```python
from build123d import *

# Parameters (mm, degrees)
SKETCH1_W           = 234
SKETCH1_H           = 178
BOSS_EXTRUDE1_DEPTH = 3
BOSS_EXTRUDE1_TAPER = 9
SKETCH2_R           = 3.5
SKETCH2_R_2         = 1.4
BOSS_EXTRUDE2_DEPTH = 5
SKETCH3_R           = 1.6
CUT_EXTRUDE1_DEPTH  = 3
CHAMFER1_SIZE       = 2


with BuildPart() as part:
    # Sketch1 → Boss-Extrude1 (new body)
    with BuildSketch(Plane(origin=(0, 0, 0), x_dir=(0, 0, -1), z_dir=(1, 0, 0))):
        Rectangle(SKETCH1_W, SKETCH1_H)
    extrude(amount=BOSS_EXTRUDE1_DEPTH, taper=BOSS_EXTRUDE1_TAPER)

    # Sketch2 → Boss-Extrude2 (add)
    with BuildSketch(Plane(origin=(3, 0, 0), x_dir=(0, 0, -1), z_dir=(1, 0, 0))):
        with Locations((-92.524846679, -22.175153321)):
            Circle(SKETCH2_R)
        with Locations((-92.524846679, -22.175153321)):
            Circle(SKETCH2_R_2, mode=Mode.SUBTRACT)
        with Locations((58.475153321, 62.224846679)):
            Circle(SKETCH2_R)
        with Locations((58.475153321, 62.224846679)):
            Circle(SKETCH2_R_2, mode=Mode.SUBTRACT)
        with Locations((-81.563741741, 52.524846679)):
            Circle(SKETCH2_R)
        with Locations((-81.563741741, 52.524846679)):
            Circle(SKETCH2_R_2, mode=Mode.SUBTRACT)
        with Locations((17.436258259, 52.524846679)):
            Circle(SKETCH2_R)
        with Locations((17.436258259, 52.524846679)):
            Circle(SKETCH2_R_2, mode=Mode.SUBTRACT)
        with Locations((42.436258259, 47.531127093)):
            Circle(SKETCH2_R)
        with Locations((42.436258259, 47.531127093)):
            Circle(SKETCH2_R_2, mode=Mode.SUBTRACT)
        with Locations((68.436258259, 47.531127093)):
            Circle(SKETCH2_R)
        with Locations((68.436258259, 47.531127093)):
            Circle(SKETCH2_R_2, mode=Mode.SUBTRACT)
        with Locations((42.436258259, -10.468872907)):
            Circle(SKETCH2_R)
        with Locations((42.436258259, -10.468872907)):
            Circle(SKETCH2_R_2, mode=Mode.SUBTRACT)
        with Locations((68.436258259, -10.468872907)):
            Circle(SKETCH2_R)
        with Locations((68.436258259, -10.468872907)):
            Circle(SKETCH2_R_2, mode=Mode.SUBTRACT)
        with Locations((17.436258259, 4.524846679)):
            Circle(SKETCH2_R)
        with Locations((17.436258259, 4.524846679)):
            Circle(SKETCH2_R_2, mode=Mode.SUBTRACT)
        with Locations((-81.563741741, 4.524846679)):
            Circle(SKETCH2_R)
        with Locations((-81.563741741, 4.524846679)):
            Circle(SKETCH2_R_2, mode=Mode.SUBTRACT)
        with Locations((-59.964914916, -54)):
            Circle(SKETCH2_R)
        with Locations((-59.964914916, -54)):
            Circle(SKETCH2_R_2, mode=Mode.SUBTRACT)
    extrude(amount=BOSS_EXTRUDE2_DEPTH)

    # Sketch3 → Cut-Extrude1 (cut)
    with BuildSketch(Plane.ZY):
        with Locations((-112, 84)):
            Circle(SKETCH3_R)
        with Locations((-56, 84)):
            Circle(SKETCH3_R)
        with Locations((0, 84)):
            Circle(SKETCH3_R)
        with Locations((56, 84)):
            Circle(SKETCH3_R)
        with Locations((112, 84)):
            Circle(SKETCH3_R)
        with Locations((112, 42)):
            Circle(SKETCH3_R)
        with Locations((112, 0)):
            Circle(SKETCH3_R)
        with Locations((112, -42)):
            Circle(SKETCH3_R)
        with Locations((112, -84)):
            Circle(SKETCH3_R)
        with Locations((56, -84)):
            Circle(SKETCH3_R)
        with Locations((0, -84)):
            Circle(SKETCH3_R)
        with Locations((-56, -84)):
            Circle(SKETCH3_R)
        with Locations((-112, -84)):
            Circle(SKETCH3_R)
        with Locations((-112, 42)):
            Circle(SKETCH3_R)
        with Locations((-112, 0)):
            Circle(SKETCH3_R)
        with Locations((-112, -42)):
            Circle(SKETCH3_R)
    extrude(amount=-CUT_EXTRUDE1_DEPTH, mode=Mode.SUBTRACT)

    # Chamfer1
    chamfer1_edges = [part.edges().sort_by_distance(p)[0] for p in [
        (0, 84, 54.4),
        (0, 84, -1.6),
        (0, 84, -57.6),
        (0, 84, 110.4),
        (0, -42, 110.4),
        (0, 0, 110.4),
        (0, 42, 110.4),
        (0, -84, 110.4),
        (0, -84, 54.4),
        (0, -84, -1.6),
        (0, -84, -57.6),
        (0, -84, -113.6),
        (0, 42, -113.6),
        (0, 0, -113.6),
        (0, -42, -113.6),
        (0, 84, -113.6),
    ]]
    chamfer(chamfer1_edges, length=CHAMFER1_SIZE)


solid = part.part
```
Part model, mm, in its own coordinate system. A direction names the side the tool comes from. Give positions to 0.01 mm unless a question says otherwise; leave off trailing zeros. Use CSV: the item, a comma, the result in double quotes.
Item 1: Slice it at A-A on x = 4.5. State how many separate pieces and enclosed holes the cut face has, plus the area to 3 significant figures.
Taken from the geometry:
separate pieces,"11"
enclosed holes,"11"
area,"356 mm²"
Item 2: Pin check, flat tips, straight feed: P1, Ø5, axis at y = -42, z = 112, coming from the -X side; P2, Ø1.5, axis at x = 1, y = 58.5, coming from the -Z side; P3, Ø2.5, axis at y = 84, z = -112, coming from the -X side; P4, Ø1, axis at x = 2.5, z = -61.5, coming from the -Y side. Stop position of each tip, or through.
Taken from the geometry:
P1,"stops at x = 1.1"
P2,"stops at z = -116.96"
P3,"passes through"
P4,"stops at y = -88.68"
Item 3: Which spindle directions (+Z, -Z, +X, -X, +Y, -Y) get a long thin tool onto all of the face, cutting with end or side? Do faces 4 (the face through (8, 46, -68)), 5 (the face through (5.465, 60.095, -55.698)). Say none if no direction does.
Taken from the geometry:
face 4,"+Z, -Z, +X, +Y, -Y"
face 5,"+X"
Item 4: Pull direction Y, two halves, no side cores. Call faces 1 (the face through (5.465, 3.184, 78.331)), 2 (the face through (8, -12, -68)), 3 (the face through (5.46, -51.05, 58.08)): +Y half, -Y half, draft (parallel to the pull), parting line (faces both ways), or undercut.
Taken from the geometry:
face 1,"undercut"
face 2,"draft"
face 3,"parting line"
Item 5: Drill centre lines: probe 1 along Y at (x, z) = (2.7, 112); probe 2 along Z at (x, y) = (2.7, -84); probe 3 along Y at (x, z) = (2.65, -56). Where is each one in solid material? Low to high.
Taken from the geometry:
probe 1,"y = -88.57 to -85.6, -82.4 to -43.6, -40.4 to -1.6, 1.6 to 40.4, 43.6 to 82.4, 85.6 to 88.57"
probe 2,"z = -116.57 to -113.6, -110.4 to -57.6, -54.4 to -1.6, 1.6 to 54.4, 57.6 to 110.4, 113.6 to 116.57"
probe 3,"y = -88.58 to -85.6, -82.4 to 82.4, 85.6 to 88.58"
